Source: CAD feature listing. Evaluate the final solid. Frame: model axes, mm. Coordinates: 2 decimals unless noted, no trailing zeros. Write each loop counter-clockwise with the first axis right and the second up, starting at its lowest first coordinate (ties: lowest second). Pieces come first, ordered by that corner, then holes. Notation, with made-up numbers: (-12, 63) -> (23, 63) arc R30 ccw to (23, 88) -> close; hole circle Ø5 at (45.5, 0.5). An arc over 180 degrees is marked (long way). Write item = value, one per line.
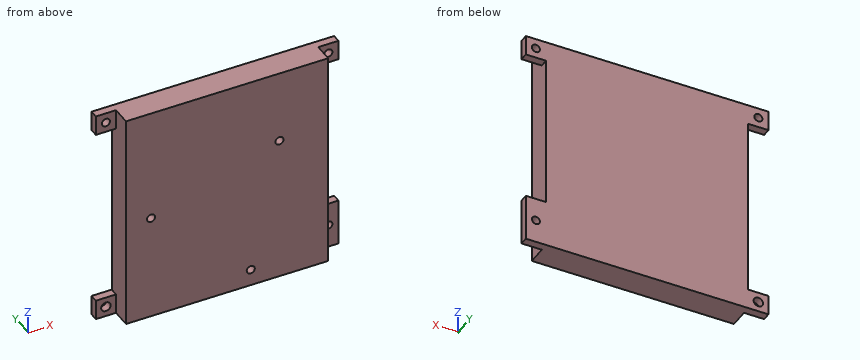
from build123d import *

# Parameters (mm, degrees)
SKETCH_1_W          = 150
SKETCH_1_H          = 165
EXTRUDE_1_DEPTH     = 20
SKETCH_2_W          = 15
SKETCH_2_H          = 15
SKETCH_2_R          = 3.5
SKETCH_2_H_2        = 34.926404716
SKETCH_2_R_2        = 3
EXTRUDE_2_DEPTH     = 6
SKETCH_4_R          = 3
CUT_EXTRUDE_1_DEPTH = 15


with BuildPart() as part:
    # Эскиз1 → Бобышка-Вытянуть1 (new body)
    with BuildSketch(Plane(origin=(0, 0, 0), x_dir=(1, 0, 0), z_dir=(0, 1, 0))):
        with Locations((124.999768599, -49.470063243)):
            Rectangle(SKETCH_1_W, SKETCH_1_H)
    extrude(amount=-EXTRUDE_1_DEPTH)

    # Эскиз2 → Бобышка-Вытянуть2 (add)
    # profile 1 of 4: a face of its own
    with BuildSketch(Plane(origin=(0, 0, 0), x_dir=(1, 0, 0), z_dir=(0, 1, 0))):
        with Locations((42.499768599, 25.529936757)):
            Rectangle(SKETCH_2_W, SKETCH_2_H)
        with Locations(Location((42.499768599, 25.529936757, 0), (0, 0, 270))):
            Circle(SKETCH_2_R, mode=Mode.SUBTRACT)
    # profile 2 of 4: a face of its own
    with BuildSketch(Plane(origin=(0, 0, 0), x_dir=(1, 0, 0), z_dir=(0, 1, 0))):
        with Locations((207.499768599, 15.566734399)):
            Rectangle(SKETCH_2_W, SKETCH_2_H_2)
        with Locations(Location((207.499768599, 15.566734399, 0), (0, 0, 270))):
            Circle(SKETCH_2_R_2, mode=Mode.SUBTRACT)
    # profile 3 of 4: a face of its own
    with BuildSketch(Plane(origin=(0, 0, 0), x_dir=(1, 0, 0), z_dir=(0, 1, 0))):
        with Locations((207.499768599, -124.470063243)):
            Rectangle(SKETCH_2_W, SKETCH_2_H)
        with Locations(Location((207.499768599, -124.470063243, 0), (0, 0, 270))):
            Circle(SKETCH_2_R_2, mode=Mode.SUBTRACT)
    # profile 4 of 4: a face of its own
    with BuildSketch(Plane(origin=(0, 0, 0), x_dir=(1, 0, 0), z_dir=(0, 1, 0))):
        with Locations((42.499768599, -124.470063243)):
            Rectangle(SKETCH_2_W, SKETCH_2_H)
        with Locations(Location((42.499768599, -124.470063243, 0), (0, 0, 270))):
            Circle(SKETCH_2_R_2, mode=Mode.SUBTRACT)
    extrude(amount=-EXTRUDE_2_DEPTH)

    # Эскиз4 → Вырез-Вытянуть1 (cut)
    with BuildSketch(Plane.XZ.offset(20)):
        with Locations(Location((163.836550468, 77.190523299, 0), (0, 0, 270))):
            Circle(SKETCH_4_R)
        with Locations(Location((142.578381334, -20.523806485, 0), (0, 0, 270))):
            Circle(SKETCH_4_R)
        with Locations(Location((68.584373995, 46.743472914, 0), (0, 0, 270))):
            Circle(SKETCH_4_R)
    extrude(amount=-CUT_EXTRUDE_1_DEPTH, mode=Mode.SUBTRACT)


solid = part.part
1) Cut plane B-B, the plane z = 38.5. Output: boundary loops of the cut face in (x, y), and give its area (3 significant figures).
Answer block:
outline = (50, -20) -> (200, -20) -> (200, 0) -> (50, 0) -> close
area = 3,000 mm2
2) Cut plane A-A, the plane x = 48. Output: boundary loops of the cut face in (y, z), and give its area (3 significant figures).
Answer block:
outline = (-6, -33.03) -> (0, -33.03) -> (0, -18.03) -> (-6, -18.03) -> close; (-6, 116.97) -> (0, 116.97) -> (0, 131.97) -> (-6, 131.97) -> close
area = 180 mm2
3) Material intervals for probe 1 along X at (y, z) = (-4, 90.5); probe 2 along X at (y, z) = (-17.5, 78.5), sorted ascending. Write a range as [from, to].
Answer block:
probe_1 = [50, 200]
probe_2 = [50, 161.14], [166.54, 200]
4) First-contact query: pin 1 Ø1.8 at (x, z) = (163.5, 75.5) entering from -Y; pin 2 Ø4.5 at (x, z) = (45, 124) entering from -Y; pin 3 Ø3 at (y, z) = (-12, 97.5) entering from +X; pin 4 Ø5.5 at (x, z) = (42.5, 124.47) entering from -Y. Flat tips, straight axial feed; report the tip coordinate or a pass-through.
Answer block:
pin_1 = -5
pin_2 = -6
pin_3 = 200
pin_4 = through
5) Cut plane C-C, the plane y = -2.5. Output: boundary loops of the cut face in (x, z), and give its area (3 significant figures).
Answer block:
outline = (35, -33.03) -> (215, -33.03) -> (215, 1.9) -> (200, 1.9) -> (200, 116.97) -> (215, 116.97) -> (215, 131.97) -> (35, 131.97) -> (35, 116.97) -> (50, 116.97) -> (50, -18.03) -> (35, -18.03) -> close; hole circle Ø7 at (42.5, -25.53); hole circle Ø6 at (42.5, 124.47); hole circle Ø6 at (207.5, -15.57); hole circle Ø6 at (207.5, 124.47)
area = 25,800 mm2
